```python
from build123d import *

# Parameters (mm, degrees)
F0_W     = 79.9999842666
F0_H     = 60
F0_W_2   = 80.0000157334
F1_DEPTH = 15
F2_R     = 57.5
F3_DEPTH = 3
F3_TAPER = -5
F4_W     = 11.6479038
F4_H     = 27.360801585
F4_W_2   = 11
F4_H_2   = 11
F4_H_3   = 24.5545655489
F5_DEPTH = 3
F6_DEPTH = 40
F9_DEPTH = 11.6479038


with BuildPart() as f1:
    # F0 (on Top) → F1 (new body)
    with BuildSketch(Plane.XY):
        with Locations((-39.9999921333, 28.1481473105)):
            Rectangle(F0_W, F0_H)
        with Locations((40.0000078667, 28.1481473105)):
            Rectangle(F0_W_2, F0_H)
        with Locations((40.0000078667, -31.8518526895)):
            Rectangle(F0_W_2, F0_H)
        with Locations((-39.9999921333, -31.8518526895)):
            Rectangle(F0_W, F0_H)
    extrude(amount=-F1_DEPTH)

    # F2 (on Top) → F3 (cut)
    with BuildSketch(Plane.XY):
        Circle(F2_R)
    extrude(amount=-F3_DEPTH, taper=F3_TAPER, mode=Mode.SUBTRACT)

    # F4 (on Top) → F5 (cut)
    with BuildSketch(Plane.XY):
        with Locations((-63.3739519, 24.3791765533)):
            Rectangle(F4_W, F4_H)
        with Locations((-63.05, -0.5552865867)):
            Rectangle(F4_W_2, F4_H_2)
        with Locations((-63.05, -22.6252786815)):
            Rectangle(F4_W_2, F4_H_3)
        with Locations((63.05, -0.5552865867)):
            Rectangle(F4_W_2, F4_H_2)
    extrude(amount=-F5_DEPTH, mode=Mode.SUBTRACT)

    # F6 (add): faces of the model
    f6_faces = [f1.faces().sort_by_distance(p)[0] for p in [
        (-63.3739519, 24.3791765533, -3),
        (-63.05, -22.6252786815, -3),
    ]]
    extrude(f6_faces, amount=F6_DEPTH)

    # F8 (on offset) → F9 (cut, through all)
    with BuildSketch(Plane.YZ.offset(-57.55)):
        Polygon((37.8841944039, 37.358019501), (10.5233872309, 37.358019501), (10.5233872309, 0), align=None)
    extrude(amount=-F9_DEPTH, mode=Mode.SUBTRACT)


solid = f1.part
```
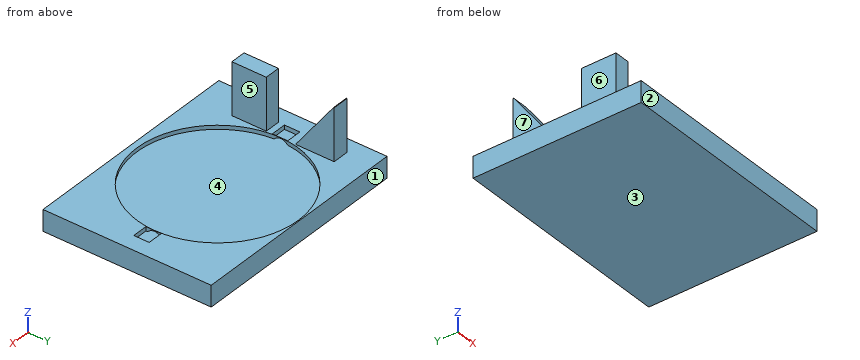
Here's how the part is built. I have some questions about the finished solid (model axes, mm). Face numbers are marked on the shaded views. A direction names the side the tool comes from. Round coordinates to 2 decimals unless told otherwise and drop trailing zeros. Loops run counter-clockwise (first coordinate to the right, second up) from the corner with the lowest first, then second, coordinate; pieces in that order, holes last.
1. Thinking about a two-plate mould opening in Y: for the marked faces 1, 2, 3 and 4, which applies, released by +Y, released by -Y, zero draft, split by the parting line, or undercut?
Answers:
face 1: released by +Y
face 2: released by -Y
face 3: zero draft
face 4: undercut
2. For the marked faces 5, 6 and 7, which set-ups out of +Z, -Z, +X, -X, +Y, -Y let a thin tool reach every point of the face, with its end or its side?
Answers:
face 5: +Z, +X, +Y, -Y
face 6: +Z, -X, -Y
face 7: +Z, -X, +Y, -Y
3. Suppose I cut it at B-B, the plane z = 21. Please give me the cut outline in (x, y), and give its area (3 significant figures).
Answers:
outline: (-69.2, 25.9) - (-57.55, 25.9) - (-57.55, 38.06) - (-69.2, 38.06) - close; (-68.55, -34.9) - (-57.55, -34.9) - (-57.55, -10.35) - (-68.55, -10.35) - close
area: 412 mm2
4. Suppose I cut it at C-C, the plane y = 3. Give the number of separate pieces and of enclosed holes in the cut face, and give its area (3 significant figures).
Answers:
separate pieces: 3
enclosed holes: 0
area: 1,990 mm2
5. Suppose I cut it at A-A, the plane x = 0. Please give me the cut outline in (y, z), and give its area (3 significant figures).
Answers:
outline: (-61.85, -15) - (58.15, -15) - (58.15, 0) - (57.5, 0) - (57.76, -3) - (-57.76, -3) - (-57.5, 0) - (-61.85, 0) - close
area: 1,450 mm2
6. Will these pins go through, and if not, where does the flat tip stop? pin 1 (3 mm diameter, centred on x = -41, z = 3, fed in from -Y); pin 2 (2 mm diameter, centred on x = -19.5, y = 18.5, fed in from +Z); pin 3 (3 mm diameter, centred on y = 12.5, z = 4.5, fed in from -X); pin 4 (5.5 mm diameter, centred on x = -65, z = 13.5, fed in from -Y).
Answers:
pin 1: passes through
pin 2: stops at z = -3
pin 3: stops at x = -69.2
pin 4: stops at y = -34.9
7. Suppose I cut it at D-D, the plane x = -61.5. Please give me the cut outline in (y, z).
Answers:
outline: (-61.85, -15) - (58.15, -15) - (58.15, 0) - (38.06, 0) - (38.06, 37) - (37.62, 37) - (10.7, 0.24) - (10.7, 0) - (4.94, 0) - (4.94, -3) - (-6.06, -3) - (-6.06, 0) - (-10.35, 0) - (-10.35, 37) - (-34.9, 37) - (-34.9, 0) - (-61.85, 0) - close
8. If I drill on probe 1 along Z at (x, y) = (51, 4.5); probe 2 along Z at (x, y) = (72, 28); probe 3 along X at (y, z) = (-30, 10), over which ranges is the centre line in solid material (lowest first)?
Answers:
probe 1: z = -15 to -3
probe 2: z = -15 to 0
probe 3: x = -68.55 to -57.55
